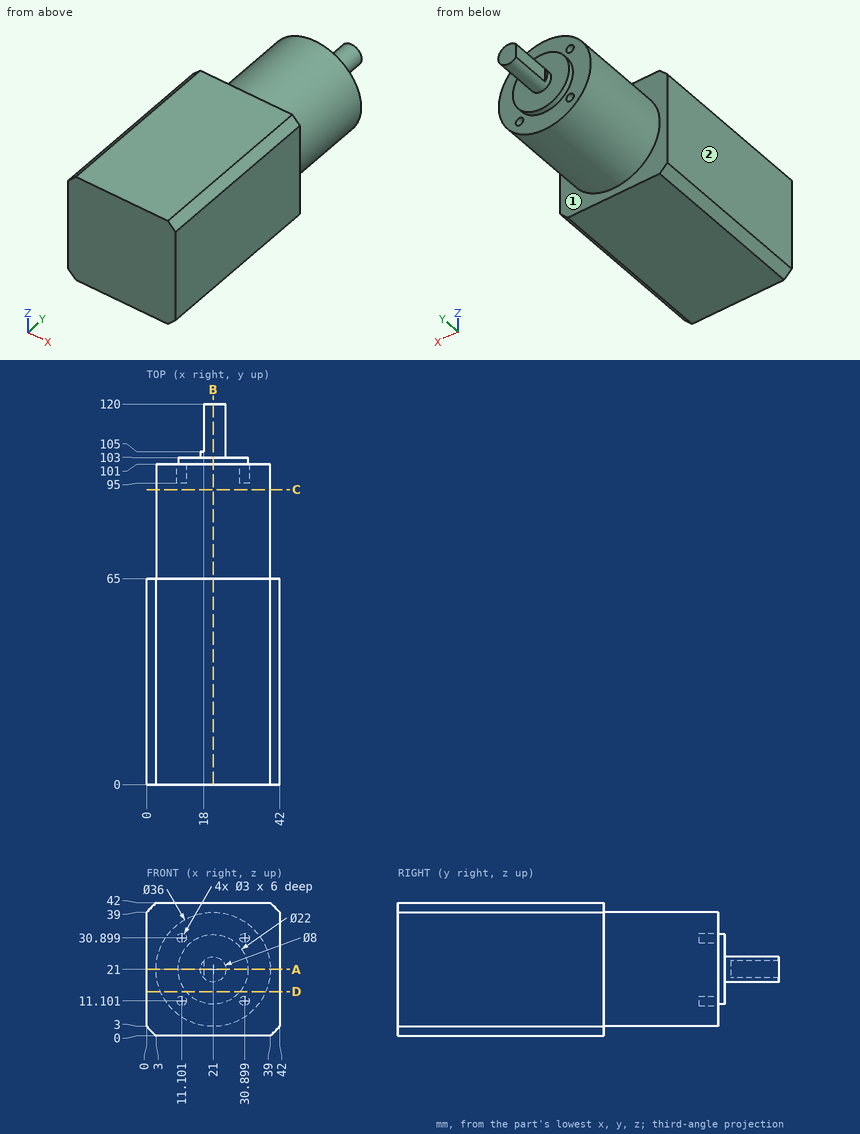
Design review of the part shown in the three views and the two pictorial views. Dimensions are in mm from the part's minimum x, y and z. A direction names the side the tool comes from. Coordinates: 2 decimals unless noted, no trailing zeros. Order: outer loops, then holes, each group sorted by start corner. A loop starts at its lowest first (then second) coordinate and runs counter-clockwise, first axis right, second up. Notation, with made-up numbers: (-3.75, 49.5) -> (18.25, 49.5) arc R18 cw to (18.25, 56.5) -> close; hole circle Ø3 at (56.25, 44). An arc over 180 degrees is marked (long way). Use one line per item in the form item = value. Start each with the question number.
(1) For probe 1 along Y at (x, z) = (33.5, 3.5); probe 2 along Y at (x, z) = (28.5, 30.5); probe 3 along X at (y, z) = (78, 9) (1 decimal), list the stretches that pass through material, from the lowest coordinate up.
(2) For the marked faces 1 and 2, list the 3-axis set-ups (+Z, -Z, +X, -X, +Y, -Y) from which the entire face can be reached by the end or side of a thin tool; tool diameter is ignored.
(3) Add section A-A on z = 21. State the section outline as (x, y) points, plus the area to 3 significant figures.
(4) Add section B-B on x = 21. State the section outline as (y, z) points, plus the area to 3 significant figures.
(5) Insertion check: pin 1 (1.5 mm diameter, centred on x = 30.5, z = 30.5, fed in from +Y); pin 2 (3.5 mm diameter, centred on x = 11, z = 11, fed in from +Y); pin 3 (1.6 mm diameter, centred on y = 109, z = 21, fed in from -X). Each pin has a flat end and moves straight along its axis. Give the tip position at first contact, or say it passes through.
(6) Add section D-D on z = 14. State the section outline as (x, y) points (1 decimal).
(7) Add section C-C on y = 93. State the section outline as (x, z) points, plus the area to 3 significant figures.
Answer block:
q1.probe_1 = 0 to 65
q1.probe_2 = 0 to 101
q1.probe_3 = 7.6 to 34.4
q2.face_1 = +Y
q2.face_2 = +Z, -Z, -X, +Y, -Y
q3.outline = (0, 0) -> (42, 0) -> (42, 65) -> (39, 65) -> (39, 101) -> (32, 101) -> (32, 103) -> (25, 103) -> (25, 120) -> (18, 120) -> (18, 105) -> (17, 105) -> (17, 103) -> (10, 103) -> (10, 101) -> (3, 101) -> (3, 65) -> (0, 65) -> close
q3.area = 4,190 mm²
q4.outline = (0, 0) -> (65, 0) -> (65, 3) -> (101, 3) -> (101, 10) -> (103, 10) -> (103, 17) -> (120, 17) -> (120, 25) -> (103, 25) -> (103, 32) -> (101, 32) -> (101, 39) -> (65, 39) -> (65, 42) -> (0, 42) -> close
q4.area = 4,210 mm²
q5.pin_1 = 95
q5.pin_2 = 101
q5.pin_3 = 18
q6.outline = (0, 0) -> (42, 0) -> (42, 65) -> (37.6, 65) -> (37.6, 101) -> (29.5, 101) -> (29.5, 103) -> (12.5, 103) -> (12.5, 101) -> (4.4, 101) -> (4.4, 65) -> (0, 65) -> close
q7.outline = circle Ø36 at (21, 21)
q7.area = 1,020 mm²
